from build123d import *

# Parameters (mm, degrees)
SKETCH1_W               = 34
SKETCH1_H               = 35.6
BOSS_EXTRUDE1_DEPTH     = 2.2
BOSS_EXTRUDE2_DEPTH     = 3
BOSS_EXTRUDE3_START     = -32
BOSS_EXTRUDE3_DEPTH     = 2
SKETCH4_R               = 2.5
SKETCH4_R_2             = 1.5
CUT_EXTRUDE1_DEPTH      = 12
SKETCH4_3_R             = 10.925
SKETCH4_3_R_2           = 1.5
SKETCH4_3_R_3           = 2.5
CUT_EXTRUDE2_DEPTH      = 2.2
SKETCH5_R               = 4
CUT_EXTRUDE3_DEPTH      = 12.2
CUT_EXTRUDE4_DEPTH      = 46.107427326
CUT_EXTRUDE4_DEPTH_BACK = 46.107427326
SKETCH6_R               = 7.5


with BuildPart() as part:
    # Sketch1 → Boss-Extrude1 (new body)
    with BuildSketch(Plane(origin=(0, 0, 0), x_dir=(1, 0, 0), z_dir=(0, 1, 0))):
        Rectangle(SKETCH1_W, SKETCH1_H)
    extrude(amount=BOSS_EXTRUDE1_DEPTH)

    # Sketch3 → Boss-Extrude2 (add)
    with BuildSketch(Plane.ZY.offset(17)):
        with BuildLine():
            Line((0, 37.8), (0, 2.2))
            Line((0, 2.2), (17.8, 2.2))
            Line((17.8, 2.2), (17.8, 20))
            ThreePointArc((17.8, 20), (12.586500705, 32.586500705), (0, 37.8))
        make_face()
        with BuildLine():
            Line((-17.8, 2.2), (0, 2.2))
            Line((0, 2.2), (0, 37.8))
            ThreePointArc((0, 37.8), (-12.586500705, 32.586500705), (-17.8, 20))
            Line((-17.8, 20), (-17.8, 2.2))
        make_face()
    extrude(amount=-BOSS_EXTRUDE2_DEPTH)

    # Sketch3<4> → Boss-Extrude3 (add)
    with BuildSketch(Plane.ZY.offset(17).offset(BOSS_EXTRUDE3_START)):
        with BuildLine():
            Line((-17.8, 2.2), (0, 2.2))
            Line((0, 2.2), (0, 37.8))
            ThreePointArc((0, 37.8), (-12.586500705, 32.586500705), (-17.8, 20))
            Line((-17.8, 20), (-17.8, 2.2))
        make_face()
        with BuildLine():
            Line((0, 37.8), (0, 2.2))
            Line((0, 2.2), (17.8, 2.2))
            Line((17.8, 2.2), (17.8, 20))
            ThreePointArc((17.8, 20), (12.586500705, 32.586500705), (0, 37.8))
        make_face()
    extrude(amount=-BOSS_EXTRUDE3_DEPTH)

    # Sketch4 → Cut-Extrude1 (cut)
    with BuildSketch(Plane.ZY.offset(17)):
        with Locations((0, 20)):
            Circle(SKETCH4_R)
        with Locations((7, 20)):
            Circle(SKETCH4_R_2)
        with Locations((0, 27)):
            Circle(SKETCH4_R_2)
        with Locations((-7, 20)):
            Circle(SKETCH4_R_2)
        with Locations((0, 13)):
            Circle(SKETCH4_R_2)
    extrude(amount=-CUT_EXTRUDE1_DEPTH, mode=Mode.SUBTRACT)

    # Sketch4<3> → Cut-Extrude2 (cut)
    with BuildSketch(Plane.ZY.offset(17)):
        with Locations((0, 20)):
            Circle(SKETCH4_3_R)
        with Locations((0, 27)):
            Circle(SKETCH4_3_R_2, mode=Mode.SUBTRACT)
        with Locations((0, 13)):
            Circle(SKETCH4_3_R_2, mode=Mode.SUBTRACT)
        with Locations((-7, 20)):
            Circle(SKETCH4_3_R_2, mode=Mode.SUBTRACT)
        with Locations((7, 20)):
            Circle(SKETCH4_3_R_2, mode=Mode.SUBTRACT)
        with Locations((0, 20)):
            Circle(SKETCH4_3_R_3, mode=Mode.SUBTRACT)
    extrude(amount=-CUT_EXTRUDE2_DEPTH, mode=Mode.SUBTRACT)

    # Sketch5 → Cut-Extrude3 (cut)
    with BuildSketch(Plane(origin=(17, 0, 0), x_dir=(0, 0, -1), z_dir=(1, 0, 0))):
        with Locations((0, 20)):
            Circle(SKETCH5_R)
    extrude(amount=-CUT_EXTRUDE3_DEPTH, mode=Mode.SUBTRACT)

    # Sketch6 → Cut-Extrude4 (cut, two sides: drawn at the far end of the back side and taken through both)
    with BuildSketch(Plane.XZ.offset(-CUT_EXTRUDE4_DEPTH_BACK)):
        with Locations(Location((0, 0, 0), (0, 0, 270))):
            Circle(SKETCH6_R)
    extrude(amount=CUT_EXTRUDE4_DEPTH + CUT_EXTRUDE4_DEPTH_BACK, mode=Mode.SUBTRACT)


solid = part.part
For this review, take the finished solid that the model builds, in its own axes (mm). A direction names the side the tool comes from. Round coordinates to 2 decimals unless told otherwise and drop trailing zeros. Order: outer loops, then holes, each group sorted by start corner. A loop starts at its lowest first (then second) coordinate and runs counter-clockwise, first axis right, second up. Notation, with made-up numbers: (77.25, 83) -> (96.25, 83) arc R27 cw to (96.25, 114) -> close; hole circle Ø1 at (30, 26). An arc over 180 degrees is marked (long way). Write item = value, one per line. Start each with the question number.
1) Take a section at C-C on z = -4.5. State the section outline as (x, y) points, plus the area to 3 significant figures.
2) The part is to be moulded in two halves that separate along Z. For faces 1 (the face through (-15.915, 30.832, -1.422)), 2 (the face through (-17, 11, 8)), 3 (the face through (0, 2, 17.8)), say which applies: +Z half, -Z half, draft (parallel to the pull), parting line (faces both ways), or undercut.
3) To check wall thickness, follow line 1 (X direction, y = 11, z = 10); line 2 (X direction, y = 14.5, z = 6); line 3 (X direction, y = 20.5, z = 6.5). State the ranges of each line that lie inside material, in increasing order. Write a range as from..to.
4) Take a section at B-B on x = 0. State the section outline as (y, z) points, plus the area to 3 significant figures.
5) Take a section at A-A on y = 8. State the section outline as (x, z) points, plus the area to 3 significant figures.
6) Tool access review of faces 4 (the face through (-14.406, 11.536, -0.325)), 5 (the face through (16.014, 23.966, 0.521)), 6 (the face through (-14, 16, 0)), 7 (the face through (-8, 0, 0)): name each direction out of +Z, -Z, +X, -X, +Y, -Y from which nothing blocks a thin tool from reaching the whole face with its end or side.
7) Take a section at D-D on y = 23. State the section outline as (x, z) points, plus the area to 3 significant figures.
8) Insertion check: pin 1 (17.5 mm diameter, centred on y = 20, z = 0, fed in from -X); pin 2 (10 mm diameter, centred on x = 5.5, z = -5, fed in from +Y); pin 3 (5 mm diameter, centred on x = -9.5, y = 30.5, fed in from -Z); pin 4 (1.8 mm diameter, centred on y = 27, z = 0, fed in from -X). Each pin has a flat end and moves straight along its axis. Give the tip position at first contact, or say it passes through.
Verdict:
q1.outline = (-17, 0) -> (-6, 0) -> (-6, 2.2) -> (-14, 2.2) -> (-14, 37.22) -> (-17, 37.22) -> (-17, 29.96) -> (-14.8, 29.96) -> (-14.8, 10.04) -> (-17, 10.04) -> close; (6, 0) -> (17, 0) -> (17, 37.22) -> (15, 37.22) -> (15, 2.2) -> (6, 2.2) -> close
q1.area = 180 mm2
q2.face_1 = undercut
q2.face_2 = draft
q2.face_3 = +Z half
q3.line_1 = -17..-14, 15..17
q3.line_2 = -14.8..-14, 15..17
q3.line_3 = 15..17
q4.outline = (0, -17.8) -> (2.2, -17.8) -> (2.2, -7.5) -> (0, -7.5) -> close; (0, 7.5) -> (2.2, 7.5) -> (2.2, 17.8) -> (0, 17.8) -> close
q4.area = 45.3 mm2
q5.outline = (-17, -17.8) -> (-14, -17.8) -> (-14, 17.8) -> (-17, 17.8) -> close; (15, -17.8) -> (17, -17.8) -> (17, 17.8) -> (15, 17.8) -> close
q5.area = 178 mm2
q6.face_4 = -X
q6.face_5 = +X
q6.face_6 = +Z, -Z, +Y
q6.face_7 = +Z, -Z, +X, -X, -Y
q7.outline = (-17, -17.55) -> (-14, -17.55) -> (-14, 17.55) -> (-17, 17.55) -> (-17, 10.51) -> (-14.8, 10.51) -> (-14.8, -10.51) -> (-17, -10.51) -> close; (15, -17.55) -> (17, -17.55) -> (17, -2.65) -> (15, -2.65) -> close; (15, 2.65) -> (17, 2.65) -> (17, 17.55) -> (15, 17.55) -> close
q7.area = 119 mm2
q8.pin_1 = -14.8
q8.pin_2 = 2.2
q8.pin_3 = through
q8.pin_4 = 15
